Part model, mm, in its own coordinate system. Face numbers are marked on the shaded views. A direction names the side the tool comes from. Coordinates: 2 decimals unless noted, no trailing zeros. Write each loop counter-clockwise with the first axis right and the second up, starting at its lowest first coordinate (ties: lowest second). Pieces come first, ordered by that corner, then holes. Notation, with made-up numbers: (-39.5, 17) -> (10.5, 17) arc R24 cw to (10.5, 33) -> close; hole circle Ø2 at (80, 82). An arc over 180 degrees is marked (long way). Write item = value, one per line.
from build123d import *

# Parameters (mm, degrees)
EXTRUDE_1_DEPTH     = 30
SKETCH_3_R          = 2
CUT_EXTRUDE_2_DEPTH = 10
SKETCH_4_R          = 2
CUT_EXTRUDE_3_DEPTH = 10
SKETCH_2_R          = 1.8
CUT_EXTRUDE_4_DEPTH = 9


with BuildPart() as part:
    # 草圖1 → 填料-伸長1 (new body)
    with BuildSketch(Plane(origin=(0, 0, 0), x_dir=(1, 0, 0), z_dir=(0, 1, 0))):
        Polygon((0, 0), (0, 108.1), (80.5, 108.1), (80.5, 103.1), (8, 103.1), (8, 0), align=None)
    extrude(amount=EXTRUDE_1_DEPTH)

    # 草圖3 → 除料-伸長2 (cut)
    with BuildSketch(Plane.ZY):
        with Locations((-20, 23)):
            Circle(SKETCH_3_R)
        with Locations((-20, 15)):
            Circle(SKETCH_3_R)
        with Locations((-20, 7)):
            Circle(SKETCH_3_R)
        with Locations((-28, 23)):
            Circle(SKETCH_3_R)
        with Locations((-28, 15)):
            Circle(SKETCH_3_R)
        with Locations((-28, 7)):
            Circle(SKETCH_3_R)
        with Locations((-36, 23)):
            Circle(SKETCH_3_R)
        with Locations((-36, 15)):
            Circle(SKETCH_3_R)
        with Locations((-36, 7)):
            Circle(SKETCH_3_R)
        with Locations((-64.1, 23)):
            Circle(SKETCH_3_R)
        with Locations((-64.1, 15)):
            Circle(SKETCH_3_R)
        with Locations((-64.1, 7)):
            Circle(SKETCH_3_R)
        with Locations((-72.1, 23)):
            Circle(SKETCH_3_R)
        with Locations((-72.1, 15)):
            Circle(SKETCH_3_R)
        with Locations((-72.1, 7)):
            Circle(SKETCH_3_R)
        with Locations((-80.1, 23)):
            Circle(SKETCH_3_R)
        with Locations((-80.1, 15)):
            Circle(SKETCH_3_R)
        with Locations((-80.1, 7)):
            Circle(SKETCH_3_R)
        with Locations((-88.1, 23)):
            Circle(SKETCH_3_R)
        with Locations((-88.1, 15)):
            Circle(SKETCH_3_R)
        with Locations((-88.1, 7)):
            Circle(SKETCH_3_R)
    extrude(amount=-CUT_EXTRUDE_2_DEPTH, mode=Mode.SUBTRACT)

    # 草圖4 → 除料-伸長3 (cut)
    with BuildSketch(Plane(origin=(0, 0, -108.1), x_dir=(-1, 0, 0), z_dir=(0, 0, -1))):
        with Locations((-74.2, 26)):
            Circle(SKETCH_4_R)
        with Locations((-74.2, 18)):
            Circle(SKETCH_4_R)
        with Locations((-74.2, 10)):
            Circle(SKETCH_4_R)
    extrude(amount=-CUT_EXTRUDE_3_DEPTH, mode=Mode.SUBTRACT)

    # 草圖2 → 除料-伸長4 (cut)
    with BuildSketch(Plane.XY):
        with Locations((4, 23)):
            Circle(SKETCH_2_R)
        with Locations((4, 7)):
            Circle(SKETCH_2_R)
        with Locations((4, 15)):
            Circle(SKETCH_2_R)
    extrude(amount=-CUT_EXTRUDE_4_DEPTH, mode=Mode.SUBTRACT)


solid = part.part
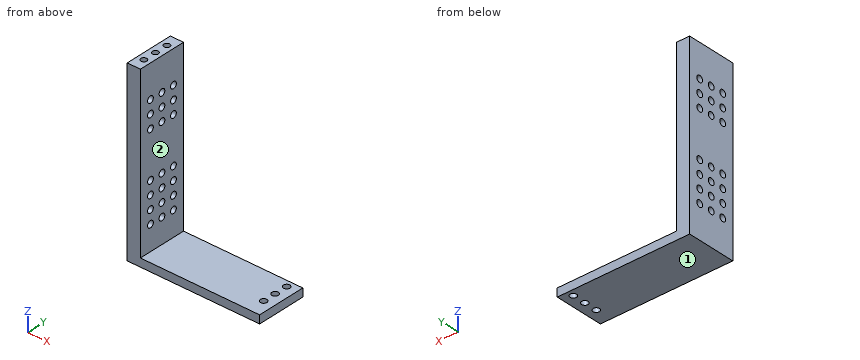
Q1. Saw through at A-A on z = -88.1. Give the cut face in (x, y), and give its area (3 significant figures).
Model answer:
outline = (0, 0) -> (8, 0) -> (8, 5) -> (0, 5) -> close; (0, 9) -> (8, 9) -> (8, 13) -> (0, 13) -> close; (0, 17) -> (8, 17) -> (8, 21) -> (0, 21) -> close; (0, 25) -> (8, 25) -> (8, 30) -> (0, 30) -> close
area = 144 mm²
Q2. Saw through at D-D on z = -52. Give the cut face in (x, y).
Model answer:
outline = (0, 0) -> (8, 0) -> (8, 30) -> (0, 30) -> close
Q3. Probe line 1 (Y direction, x = 1, z = -64); line 2 (Y direction, x = 4, z = -5); line 3 (X direction, y = 23.75, z = -48). List the from-to ranges inside material, lowest first. Write a range as from..to.
Model answer:
line_1 = 0..5, 9..13, 17..21, 25..30
line_2 = 0..5.2, 8.8..13.2, 16.8..21.2, 24.8..30
line_3 = 0..8
Q4. Saw through at B-B on x = 4. Count the separate pieces of the cut face and the enclosed holes in it, and give its area (3 significant figures).
Model answer:
separate_pieces = 1
enclosed_holes = 21
area = 2,880 mm²
Q5. Which spindle directions (+Z, -Z, +X, -X, +Y, -Y) get a long thin tool onto all of the face, cutting with end or side? Do the marked faces 1 and 2. Say none if no direction does.
Model answer:
face_1 = -Z, +X, -X, +Y, -Y
face_2 = +Z, +X, +Y, -Y
Q6. Pin check, flat tips, straight feed: pin 1 (3.5 mm diameter, centred on y = 15, z = -64.1, fed in from -X); pin 2 (6 mm diameter, centred on x = 27.5, y = 16, fed in from +Z); pin 3 (5 mm diameter, centred on y = 16.5, z = -48.5, fed in from +X). Stop position of each tip, or through.
Model answer:
pin_1 = through
pin_2 = -103.1
pin_3 = 8
Q7. Saw through at C-C on x = 32.5. Give the cut face in (y, z).
Model answer:
outline = (0, -108.1) -> (30, -108.1) -> (30, -103.1) -> (0, -103.1) -> close
